Autodesk Inventor part; units mm, degrees
ref_plane "YZ Plane" through (0, 0, 0) normal (1, 0, 0) x (0, 1, 0)
ref_plane "XZ Plane" through (0, 0, 0) normal (0, 1, 0) x (-1, 0, 0)
ref_plane "XY Plane" through (0, 0, 0) normal (0, 0, 1) x (1, 0, 0)
sketch "スケッチ1" plane through (0, 0, 0) normal (0, 1, 0) x (-1, 0, 0)
  line L0 (0, 0) -> (-38, 0)
  line L1 (-38, 0) -> (-38, -48)
  line L2 (-38, -48) -> (0, -48)
  line L3 (0, -48) -> (0, 0)
  dimension "d0" = 48
  dimension "d1" = 38
extrude "押し出し1" add sketch "スケッチ1" along normal blind 47.5
sketch "スケッチ2" plane through (38, 0, -48) normal (0, 0, -1) x (-1, 0, 0)
  line L0 (4, 43.5) -> (59.072, 43.5)
  line L1 (59.072, 43.5) -> (59.072, 4)
  line L2 (59.072, 4) -> (4, 4)
  line L3 (4, 4) -> (4, 43.5)
  line L4 (0, 47.5) -> (38, 47.5)
  line L5 (0, 0) -> (38, 0)
  line L6 (0, 0) -> (0, 47.5)
  dimension "d4" = 39.5
  dimension "d6" = 4
  dimension "d7" = 4
extrude "押し出し2" cut sketch "スケッチ2" against normal blind 100
sketch "スケッチ3" plane through (0, 47.5, 0) normal (0, 1, 0) x (1, 0, 0)
  line L0 (38, 48) -> (0, 48)
  line L1 (38, 0) -> (38, 48)
  point P0 (0, 0)
  point P1 (17, 32)
  dimension "d10" = 16
  dimension "d11" = 21
hole "穴1" at (17, 47.5, -32) direction (0, -1, 0) diameter 22 end through all
sketch "スケッチ4" plane through (0, 47.5, 0) normal (0, 1, 0) x (1, 0, 0)
  line L0 (0, 0) -> (38, 0)
  line L1 (38, 0) -> (38, 48)
  point P0 (30.5, 4)
  point P1 (30.5, 31)
  point P2 (3.5, 4)
  point P3 (3.5, 31)
  point P4 (3.5, 4)
  dimension "d19" = 4
  dimension "d20" = 7.5
  dimension "d23" = 27
  dimension "d26" = 27
hole "穴2" at (30.5, 47.5, -4) at (30.5, 47.5, -31) at (3.5, 47.5, -31) at (3.5, 47.5, -4) direction (0, -1, 0) diameter 3.2 end through all
sketch "スケッチ6" plane through (38, 0, 0) normal (1, 0, 0) x (0, 0, -1)
  line L0 (0, 47.5) -> (48, 47.5)
  line L1 (0, 0) -> (0, 47.5)
  point P0 (10, 32.5)
  point P1 (32, 32.5)
  point P2 (10, 17.5)
  point P3 (32, 17.5)
  dimension "d45" = 15
  dimension "d46" = 10
  dimension "d49" = 22
  dimension "d52" = 15
hole "穴4" at (38, 32.5, -10) at (38, 32.5, -32) at (38, 17.5, -10) at (38, 17.5, -32) direction (-1, 0, 0) diameter 1 end through all
fillet "フィレット1" radius 2 2 edges at (34, 4, -24) (34, 43.5, -24)
properties part number "サーボモータ固定２軸"
Geometry: final body of the model. Coordinates: model frame, mm. A direction names the side the tool comes from. Coordinates: 2 decimals unless noted, no trailing zeros. Loops run counter-clockwise (first coordinate to the right, second up) from the corner with the lowest first, then second, coordinate; pieces in that order, holes last. Notation, with made-up numbers: M 63,61 L 105,61 A28 cw 105,86 Z; hole C -22,82 d5. An arc over 180 degrees is marked long. Put each result on its own line as item: value.
(1) Material intervals for probe 1 along X at (y, z) = (1.75, -4); probe 2 along Y at (x, z) = (36, -32); probe 3 along Y at (x, z) = (17.5, -5.5), sorted ascending.
Answer sheet:
probe 1: x = 0 to 1.9, 5.1 to 28.9, 32.1 to 38
probe 2: y = 0 to 17, 18 to 32, 33 to 47.5
probe 3: y = 0 to 4, 43.5 to 47.5
(2) Access query for faces 1 (the face through (34, 24, -24)), 2 (the face through (0, 45, -24)). Directions: +Z, -Z, +X, -X, +Y, -Y. A direction counts if a zero-diameter tool reaches every point of the face in a straight line with its end or side. Return the directions, or none.
Answer sheet:
face 1: +Z, -Z, -X
face 2: +Z, -Z, -X, +Y, -Y
(3) Cut plane C-C on z = -45. Return the cut outline in (x, y).
Answer sheet:
outline: M 0,0 L 38,0 L 38,47.5 L 0,47.5 L 0,43.5 L 32,43.5 A2 cw 34,41.5 L 34,6 A2 cw 32,4 L 0,4 Z
(4) Cut plane A-A on x = 30.5. Return the cut outline in (y, z).
Answer sheet:
outline: M 0,-48 L 4,-48 L 4,-32.6 L 0,-32.6 Z; M 0,-29.4 L 4,-29.4 L 4,-5.6 L 0,-5.6 Z; M 0,-2.4 L 4,-2.4 L 4,0 L 0,0 Z; M 43.5,-48 L 47.5,-48 L 47.5,-32.6 L 43.5,-32.6 Z; M 43.5,-29.4 L 47.5,-29.4 L 47.5,-5.6 L 43.5,-5.6 Z; M 43.5,-2.4 L 47.5,-2.4 L 47.5,0 L 43.5,0 Z
(5) Draft query along Y for faces 3 (the face through (16, 4, -19)), 4 (the face through (19, 0, -18)), 5 (the face through (28.914, 45.472, -4.208)). Return one class per face: pulls with the +Y half, pulls with the -Y half, needs draft (parallel to the pull), parting line crosses it, or undercut.
Answer sheet:
face 3: undercut
face 4: pulls with the -Y half
face 5: needs draft
(6) Cut plane B-B on x = 17. Return the cut outline in (y, z).
Answer sheet:
outline: M 0,-48 L 4,-48 L 4,-43 L 0,-43 Z; M 0,-21 L 4,-21 L 4,0 L 0,0 Z; M 43.5,-48 L 47.5,-48 L 47.5,-43 L 43.5,-43 Z; M 43.5,-21 L 47.5,-21 L 47.5,0 L 43.5,0 Z
(7) First-contact query: pin 1 (3 mm diameter, centred on x = 30.5, z = -4, fed in from -Y); pin 2 (1 mm diameter, centred on y = 30, z = -37, fed in from -X). Flat tips, straight axial feed; report the tip coordinate or a pass-through.
Answer sheet:
pin 1: passes through
pin 2: stops at x = 34
